Geometry: final body of the model. Coordinates: model frame, mm. A direction names the side the tool comes from. Give positions to 0.01 mm unless a question says otherwise; leave off trailing zeros. Order: outer loops, then holes, each group sorted by start corner. A loop starts at its lowest first (then second) coordinate and runs counter-clockwise, first axis right, second up. Notation, with made-up numbers: (78, -25) - (132, -25) arc R15 ccw to (132, -9) - close; hole circle Ø11 at (-37, 28.5). An arc over 180 degrees is marked (long way). One line per item, written item: value.
```python
from build123d import *

# Parameters (mm, degrees)
BOSS_EXTRUDE1_DEPTH = 50


with BuildPart() as part:
    # Sketch1 → Boss-Extrude1 (new body)
    with BuildSketch(Plane.XY):
        with BuildLine():
            Line((-2.746356642, -3.807016814), (-5.847983186, -6.908643358))
            ThreePointArc((-5.847983186, -6.908643358), (-5.956791575, -7.07148662), (-5.995, -7.263573344))
            Line((-5.995, -7.263573344), (-5.995, -7.858053199))
            ThreePointArc((-5.995, -7.858053199), (-5.847983186, -8.212983186), (-5.493053199, -8.36))
            Line((-5.493053199, -8.36), (-3.131946801, -8.36))
            ThreePointArc((-3.131946801, -8.36), (-2.777016814, -8.507016814), (-2.63, -8.861946801))
            Line((-2.63, -8.861946801), (-2.63, -9.498053199))
            ThreePointArc((-2.63, -9.498053199), (-2.777016814, -9.852983186), (-3.131946801, -10))
            Line((-3.131946801, -10), (-8.5, -10))
            ThreePointArc((-8.5, -10), (-9.560660172, -9.560660172), (-10, -8.5))
            Line((-10, -8.5), (-10, -3.131946801))
            ThreePointArc((-10, -3.131946801), (-9.852983186, -2.777016814), (-9.498053199, -2.63))
            Line((-9.498053199, -2.63), (-8.861946801, -2.63))
            ThreePointArc((-8.861946801, -2.63), (-8.507016814, -2.777016814), (-8.36, -3.131946801))
            Line((-8.36, -3.131946801), (-8.36, -5.493053199))
            ThreePointArc((-8.36, -5.493053199), (-8.212983186, -5.847983186), (-7.858053199, -5.995))
            Line((-7.858053199, -5.995), (-7.263573344, -5.995))
            ThreePointArc((-7.263573344, -5.995), (-7.07148662, -5.956791575), (-6.908643358, -5.847983186))
            Line((-6.908643358, -5.847983186), (-3.807016814, -2.746356642))
            ThreePointArc((-3.807016814, -2.746356642), (-3.698208425, -2.58351338), (-3.66, -2.391426656))
            Line((-3.66, -2.391426656), (-3.66, 2.391426656))
            ThreePointArc((-3.66, 2.391426656), (-3.698208425, 2.58351338), (-3.807016814, 2.746356642))
            Line((-3.807016814, 2.746356642), (-6.908643358, 5.847983186))
            ThreePointArc((-6.908643358, 5.847983186), (-7.07148662, 5.956791575), (-7.263573344, 5.995))
            Line((-7.263573344, 5.995), (-7.858053199, 5.995))
            ThreePointArc((-7.858053199, 5.995), (-8.212983186, 5.847983186), (-8.36, 5.493053199))
            Line((-8.36, 5.493053199), (-8.36, 3.131946801))
            ThreePointArc((-8.36, 3.131946801), (-8.507016814, 2.777016814), (-8.861946801, 2.63))
            Line((-8.861946801, 2.63), (-9.498053199, 2.63))
            ThreePointArc((-9.498053199, 2.63), (-9.852983186, 2.777016814), (-10, 3.131946801))
            Line((-10, 3.131946801), (-10, 8.5))
            ThreePointArc((-10, 8.5), (-9.560660172, 9.560660172), (-8.5, 10))
            Line((-8.5, 10), (-3.131946801, 10))
            ThreePointArc((-3.131946801, 10), (-2.777016814, 9.852983186), (-2.63, 9.498053199))
            Line((-2.63, 9.498053199), (-2.63, 8.861946801))
            ThreePointArc((-2.63, 8.861946801), (-2.777016814, 8.507016814), (-3.131946801, 8.36))
            Line((-3.131946801, 8.36), (-5.493053199, 8.36))
            ThreePointArc((-5.493053199, 8.36), (-5.847983186, 8.212983186), (-5.995, 7.858053199))
            Line((-5.995, 7.858053199), (-5.995, 7.263573344))
            ThreePointArc((-5.995, 7.263573344), (-5.956791575, 7.07148662), (-5.847983186, 6.908643358))
            Line((-5.847983186, 6.908643358), (-2.746356642, 3.807016814))
            ThreePointArc((-2.746356642, 3.807016814), (-2.58351338, 3.698208425), (-2.391426656, 3.66))
            Line((-2.391426656, 3.66), (2.391426656, 3.66))
            ThreePointArc((2.391426656, 3.66), (2.58351338, 3.698208425), (2.746356642, 3.807016814))
            Line((2.746356642, 3.807016814), (5.847983186, 6.908643358))
            ThreePointArc((5.847983186, 6.908643358), (5.956791575, 7.07148662), (5.995, 7.263573344))
            Line((5.995, 7.263573344), (5.995, 7.858053199))
            ThreePointArc((5.995, 7.858053199), (5.847983186, 8.212983186), (5.493053199, 8.36))
            Line((5.493053199, 8.36), (3.131946801, 8.36))
            ThreePointArc((3.131946801, 8.36), (2.777016814, 8.507016814), (2.63, 8.861946801))
            Line((2.63, 8.861946801), (2.63, 9.498053199))
            ThreePointArc((2.63, 9.498053199), (2.777016814, 9.852983186), (3.131946801, 10))
            Line((3.131946801, 10), (8.5, 10))
            ThreePointArc((8.5, 10), (9.560660172, 9.560660172), (10, 8.5))
            Line((10, 8.5), (10, 3.131946801))
            ThreePointArc((10, 3.131946801), (9.852983186, 2.777016814), (9.498053199, 2.63))
            Line((9.498053199, 2.63), (8.861946801, 2.63))
            ThreePointArc((8.861946801, 2.63), (8.507016814, 2.777016814), (8.36, 3.131946801))
            Line((8.36, 3.131946801), (8.36, 5.493053199))
            ThreePointArc((8.36, 5.493053199), (8.212983186, 5.847983186), (7.858053199, 5.995))
            Line((7.858053199, 5.995), (7.263573344, 5.995))
            ThreePointArc((7.263573344, 5.995), (7.07148662, 5.956791575), (6.908643358, 5.847983186))
            Line((6.908643358, 5.847983186), (3.807016814, 2.746356642))
            ThreePointArc((3.807016814, 2.746356642), (3.698208425, 2.58351338), (3.66, 2.391426656))
            Line((3.66, 2.391426656), (3.66, -2.391426656))
            ThreePointArc((3.66, -2.391426656), (3.698208425, -2.58351338), (3.807016814, -2.746356642))
            Line((3.807016814, -2.746356642), (6.908643358, -5.847983186))
            ThreePointArc((6.908643358, -5.847983186), (7.07148662, -5.956791575), (7.263573344, -5.995))
            Line((7.263573344, -5.995), (7.858053199, -5.995))
            ThreePointArc((7.858053199, -5.995), (8.212983186, -5.847983186), (8.36, -5.493053199))
            Line((8.36, -5.493053199), (8.36, -3.131946801))
            ThreePointArc((8.36, -3.131946801), (8.507016814, -2.777016814), (8.861946801, -2.63))
            Line((8.861946801, -2.63), (9.498053199, -2.63))
            ThreePointArc((9.498053199, -2.63), (9.852983186, -2.777016814), (10, -3.131946801))
            Line((10, -3.131946801), (10, -8.5))
            ThreePointArc((10, -8.5), (9.560660172, -9.560660172), (8.5, -10))
            Line((8.5, -10), (3.131946801, -10))
            ThreePointArc((3.131946801, -10), (2.777016814, -9.852983186), (2.63, -9.498053199))
            Line((2.63, -9.498053199), (2.63, -8.861946801))
            ThreePointArc((2.63, -8.861946801), (2.777016814, -8.507016814), (3.131946801, -8.36))
            Line((3.131946801, -8.36), (5.493053199, -8.36))
            ThreePointArc((5.493053199, -8.36), (5.847983186, -8.212983186), (5.995, -7.858053199))
            Line((5.995, -7.858053199), (5.995, -7.263573344))
            ThreePointArc((5.995, -7.263573344), (5.956791575, -7.07148662), (5.847983186, -6.908643358))
            Line((5.847983186, -6.908643358), (2.746356642, -3.807016814))
            ThreePointArc((2.746356642, -3.807016814), (2.58351338, -3.698208425), (2.391426656, -3.66))
            Line((2.391426656, -3.66), (-2.391426656, -3.66))
            ThreePointArc((-2.391426656, -3.66), (-2.58351338, -3.698208425), (-2.746356642, -3.807016814))
        make_face()
        with BuildLine():
            ThreePointArc((-1.767678053, 0.935582333), (-2, 0), (-1.767678053, -0.935582333))
            ThreePointArc((-1.767678053, -0.935582333), (-1.834942097, -1.834942097), (-0.935582333, -1.767678053))
            ThreePointArc((-0.935582333, -1.767678053), (0, -2), (0.935582333, -1.767678053))
            ThreePointArc((0.935582333, -1.767678053), (1.834942097, -1.834942097), (1.767678053, -0.935582333))
            ThreePointArc((1.767678053, -0.935582333), (2, 0), (1.767678053, 0.935582333))
            ThreePointArc((1.767678053, 0.935582333), (1.834942097, 1.834942097), (0.935582333, 1.767678053))
            ThreePointArc((0.935582333, 1.767678053), (0, 2), (-0.935582333, 1.767678053))
            ThreePointArc((-0.935582333, 1.767678053), (-1.834942097, 1.834942097), (-1.767678053, 0.935582333))
        make_face(mode=Mode.SUBTRACT)
    extrude(amount=BOSS_EXTRUDE1_DEPTH)


solid = part.part
```
1) Set-up query: faces 1 (the face through (0, 3.66, 25)), 2 (the face through (-3.66, 0, 25)), 3 (the face through (8.36, -4, 25)). Return all of +Z, -Z, +X, -X, +Y, -Y with unobstructed straight access to the full face (end or side cutting, diameter ignored); none if empty.
Answers below:
face 1: +Z, -Z, +Y
face 2: +Z, -Z, -X
face 3: +Z, -Z
2) Section A-A, the plane x = 4.5. Return loops of the section in (y, z).
Answers below:
outline: (-10, 0) - (-8.36, 0) - (-8.36, 50) - (-10, 50) - close; (-5.56, 0) - (-3.44, 0) - (-3.44, 50) - (-5.56, 50) - close; (3.44, 0) - (5.56, 0) - (5.56, 50) - (3.44, 50) - close; (8.36, 0) - (10, 0) - (10, 50) - (8.36, 50) - close
3) First-contact query: pin 1 (2.5 mm diameter, centred on y = 0.5, z = 33.5, fed in from +X); pin 2 (0.5 mm diameter, centred on x = 9, z = 19, fed in from -Y); pin 3 (3 mm diameter, centred on y = 0.5, z = 30, fed in from -X). Flat tips, straight axial feed; report the tip coordinate or a pass-through.
Answers below:
pin 1: x = 3.66
pin 2: y = -9.98
pin 3: x = -3.66
4) Mould query, pull axis Y, two halves, no side actions, for faces 4 (the face through (1.825, -1.845, 24.65)), 5 (the face through (-4, 8.36, 25)), 6 (the face through (-9.57, 9.55, 24.65)), 7 (the face through (-10, -6, 25)). Classes: released by +Y, released by -Y, zero draft, split by the parting line, or undercut.
Answers below:
face 4: undercut
face 5: undercut
face 6: released by +Y
face 7: zero draft
5) Section B-B, the plane y = -4.75. Return loops of the section in (x, z), then the cut area to 3 significant figures.
Answers below:
outline: (-10, 0) - (-8.36, 0) - (-8.36, 50) - (-10, 50) - close; (-5.81, 0) - (-3.69, 0) - (-3.69, 50) - (-5.81, 50) - close; (3.69, 0) - (5.81, 0) - (5.81, 50) - (3.69, 50) - close; (8.36, 0) - (10, 0) - (10, 50) - (8.36, 50) - close
area: 376 mm^2
6) Material intervals for line 1 along X through (y, z) = (-3.25, 12.5); line 2 along Y through (x, z) = (5.5, 28); line 3 along X through (y, z) = (-3, 31), sorted ascending.
Answers below:
line 1: -10 to -8.36, -4.31 to 4.31, 8.36 to 10
line 2: -10 to -8.36, -6.56 to -4.44, 4.44 to 6.56, 8.36 to 10
line 3: -9.98 to -8.38, -4.06 to 4.06, 8.38 to 9.98
